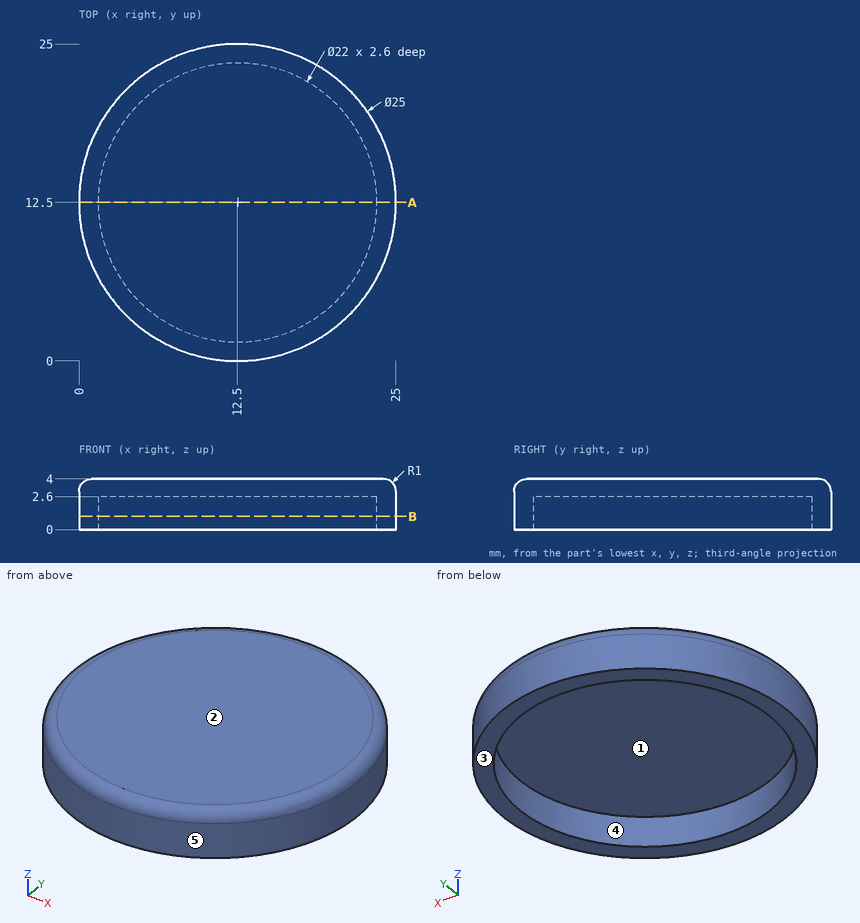
Here's the drawing with two shaded views (mm, measured from the low corner). I have some questions. A direction names the side the tool comes from. Coordinates: 2 decimals unless noted, no trailing zeros. Write each loop counter-clockwise with the first axis right and the second up, starting at its lowest first coordinate (ties: lowest second). Pieces come first, ordered by that corner, then holes. Notation, with made-up numbers: M 18.5,-24 L 46.5,-24 A31 cw 46.5,7 Z; hole C -18.75,16.25 d9. An arc over 180 degrees is marked long. Answer as CSV lines item,"result". Start each with the question number.
1) We'd pull the mould along X, two halves only. Please class the marked faces 3, 4 and 5: +X half, -X half, draft (parallel to the pull), parting line (faces both ways), or undercut.
2) I want a section at A-A, the plane y = 12.5. Please give me the cut outline in (x, z).
3) Please list where these lines run through material, in increasing order: line 1 (Y direction, x = 12.5, z = 1.65); line 2 (Z direction, x = 13.25, y = 3); line 3 (Y direction, x = 22, z = 1.85). Write a range as from..to.
4) For the marked faces 1 and 2, which set-ups out of +Z, -Z, +X, -X, +Y, -Y let a thin tool reach every point of the face, with its end or its side?
5) I want a section at B-B, the plane z = 1.05. Please give me the cut outline in (x, y).
6) For P1, Ø10, axis at x = 9.5, y = 17, coming from the -Z side; P2, Ø1, axis at x = 19.5, z = 2.5, coming from the -Y side, each with a flat end and sliding along its axis, tell me the tip position at first contact or that it passes through.
Data:
1,face 3,"draft"
1,face 4,"undercut"
1,face 5,"parting line"
2,outline,"M 0,0 L 1.5,0 L 1.5,2.6 L 23.5,2.6 L 23.5,0 L 25,0 L 25,3 A1 ccw 24,4 L 1,4 A1 ccw 0,3 Z"
3,line 1,"y = 0..1.5, 23.5..25"
3,line 2,"z = 2.6..4"
3,line 3,"y = 4.38..6.95, 18.05..20.62"
4,face 1,"-Z"
4,face 2,"+Z, +X, -X, +Y, -Y"
5,outline,"C 12.5,12.5 d25; hole C 12.5,12.5 d22"
6,P1,"stops at z = 2.6"
6,P2,"stops at y = 1.82"
